Read the model definition and answer for the solid it produces. Units are mm, in the model's axes. A direction names the side the tool comes from. Coordinates: 2 decimals unless noted, no trailing zeros. Order: outer loops, then holes, each group sorted by start corner. A loop starts at its lowest first (then second) coordinate and runs counter-clockwise, first axis right, second up. Notation, with made-up numbers: (-24.75, 76) - (9.25, 76) arc R28 ccw to (9.25, 95) - close; hole circle Ø1 at (73.5, 89.5). An arc over 180 degrees is marked (long way). Use one line per item in the form item = value. Start each with the question number.
from build123d import *

# Parameters (mm, degrees)
F0_W     = 16
F0_H     = 33.325
F0_R     = 4.1
F0_R_2   = 4.225
F0_R_3   = 1.6
F1_DEPTH = 14
F3_DEPTH = 16
F4_R     = 6


with BuildPart() as f1:
    # F0 (on Right) → F1 (new body)
    with BuildSketch(Plane.YZ):
        with Locations((8, 16.6625)):
            Rectangle(F0_W, F0_H)
        with Locations((8, 9.1)):
            Circle(F0_R, mode=Mode.SUBTRACT)
        with Locations((8, 20.1)):
            Circle(F0_R_2, mode=Mode.SUBTRACT)
        with Locations((8, 28.225)):
            Circle(F0_R_3, mode=Mode.SUBTRACT)
        with Locations((8, 20.1)):
            Circle(F0_R_2)
    extrude(amount=F1_DEPTH)

    # F2 (on face) → F3 (cut, through all)
    with BuildSketch(Plane(origin=(0, 16, 0), x_dir=(-1, 0, 0), z_dir=(0, 1, 0))):
        with BuildLine():
            ThreePointArc((-8.25, 24.135855), (-9.506928, 16.699127), (-2.775, 20.1))
            ThreePointArc((-2.775, 20.1), (-3.599127, 22.606928), (-5.75, 24.135855))
            ThreePointArc((-5.75, 24.135855), (-7, 24.325), (-8.25, 24.135855))
        make_face()
        with BuildLine():
            ThreePointArc((-8.25, 24.135855), (-7, 24.325), (-5.75, 24.135855))
            Line((-5.75, 24.135855), (-5.75, 33.325))
            Line((-5.75, 33.325), (-8.25, 33.325))
            Line((-8.25, 33.325), (-8.25, 24.135855))
        make_face()
    extrude(amount=-F3_DEPTH, mode=Mode.SUBTRACT)

    # F4
    f4_edges = [f1.edges().sort_by_distance(p)[0] for p in [
        (7, 16, 0),
        (7, 0, 0),
        (11.125, 0, 33.325),
        (2.875, 0, 33.325),
        (11.125, 16, 33.325),
        (2.875, 16, 33.325),
    ]]
    fillet(f4_edges, radius=F4_R)


solid = f1.part
Q1. A cutting plane is placed at D-D (x = 7). Give the vertices of the cut face in (y, z) (3 decimals), then the cut area to 3 significant figures.
Q2. A cutting plane is placed at C-C (x = 10). Give the vertices of the cut face in (y, z) (3 decimals), then the cut area to 3 significant figures.
Q3. A cutting plane is placed at A-A (z = 9.1). Give the vertices of the cut face in (x, y).
Q4. For a pull along Y with two mould halves and no side action, classify faces 1 (the cylindrical face through (6.9, 7.1, 5.1)), 2 (the flat face through (14, 8, 17)), 3 (the flat face through (7, 16, 14)), 4 (the cylindrical face through (7.098, 1.711, 1.804)) as +Y half, -Y half, draft (parallel to the pull), parting line (faces both ways), or undercut.
Q5. A cutting plane is placed at B-B (y = 8). Give the vertices of the cut face in (x, z) (3 decimals).
Q6. Given P1, Ø1.5, axis at x = 10, y = 2.5, coming from the +Z side, flat-ended and moving along its own axis, determine where the tip first touches the part or whether it passes through.
Q7. Consider probe 1 along Z at (x, y) = (2, 8) (3 decimals); probe 2 along X at (y, z) = (3.75, 27); probe 3 along Z at (x, y) = (5.5, 8) (3 decimals). Determine where each line is inside the solid, lowest interval first.
Q8. Which of the six approach directions +Z, -Z, +X, -X, +Y, -Y give full straight-line access (tool end or side, diameter ignored) to faces 5 (the cylindrical face through (2.92, 1.71, 31.52)), 6 (the flat face through (8.25, 6, 29))?
Result sheet:
q1.outline = (0, 6) arc R6 ccw to (6, 0) - (10, 0) arc R6 ccw to (16, 6) - (16, 15.875) - (0, 15.875) - close; hole circle Ø8.2 at (8, 9.1)
q1.area = 186 mm^2
q2.outline = (0, 6) arc R6 ccw to (6, 0) - (10, 0) arc R6 ccw to (16, 6) - (16, 17.125) - (0, 17.125) - close; (0, 23.075) - (16, 23.075) - (16, 27.325) arc R6 ccw to (10, 33.325) - (6, 33.325) arc R6 ccw to (0, 27.325) - close; hole circle Ø8.2 at (8, 9.1); hole circle Ø3.2 at (8, 28.225)
q2.area = 346 mm^2
q3.outline = (0, 0) - (14, 0) - (14, 3.9) - (0, 3.9) - close; (0, 12.1) - (14, 12.1) - (14, 16) - (0, 16) - close
q4.face_1 = undercut
q4.face_2 = draft
q4.face_3 = +Y half
q4.face_4 = -Y half
q5.outline = (0, 0) - (14, 0) - (14, 5) - (0, 5) - close; (0, 13.2) - (14, 13.2) - (14, 26.625) - (8.25, 26.625) - (8.25, 24.136) arc R4.225 cw (long way) to (5.75, 24.136) - (5.75, 26.625) - (0, 26.625) - close; (0, 29.825) - (5.75, 29.825) - (5.75, 33.325) - (0, 33.325) - close; (8.25, 29.825) - (14, 29.825) - (14, 33.325) - (8.25, 33.325) - close
q6.P1 = 32.66
q7.probe_1 = 0 to 5, 13.2 to 26.625, 29.825 to 33.325
q7.probe_2 = 0 to 5.75, 8.25 to 14
q7.probe_3 = 0 to 5, 13.2 to 16.15, 24.05 to 26.625, 29.825 to 33.325
q8.face_5 = +Z, +X, -X, -Y
q8.face_6 = +Z, +Y, -Y
